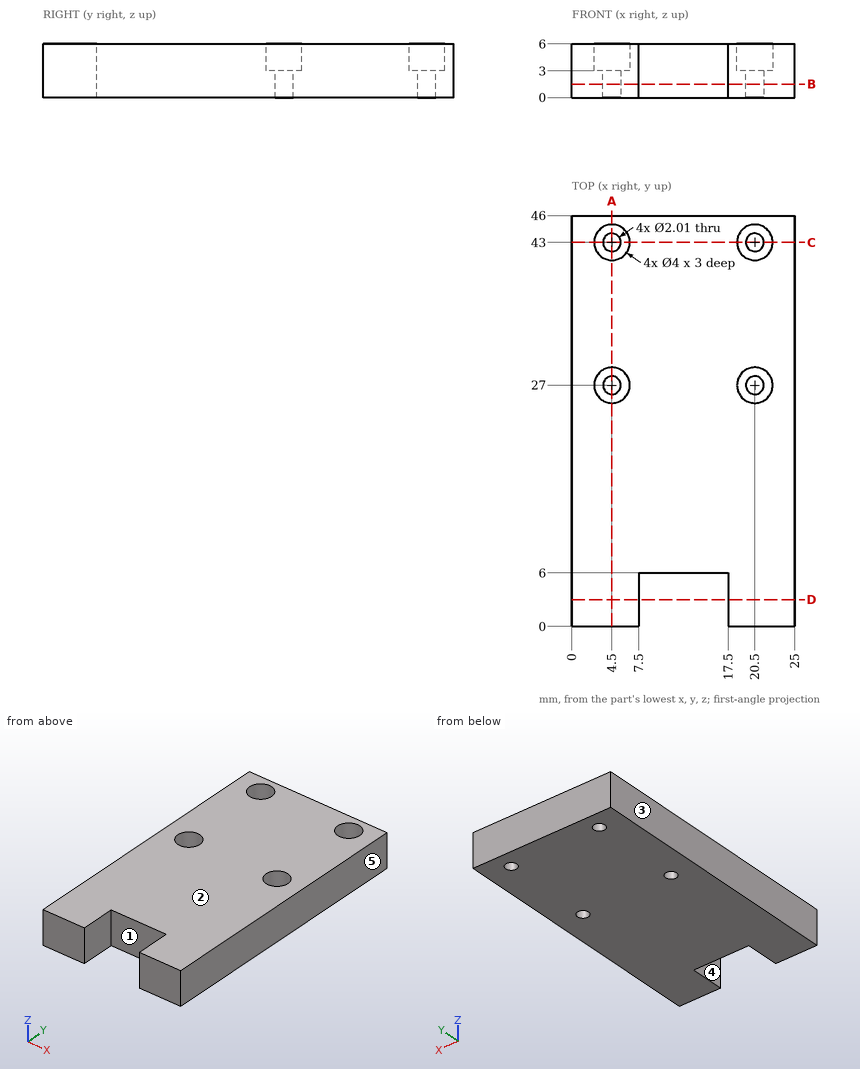
Verification items for this drawing (mm, ordinates from the low corner). A direction names the side the tool comes from. Round coordinates to 2 decimals unless told otherwise and drop trailing zeros. Loops run counter-clockwise (first coordinate to the right, second up) from the corner with the lowest first, then second, coordinate; pieces in that order, holes last. Notation, with made-up numbers: (-26, 19) -> (18, 19) arc R20 cw to (18, 58) -> close; hole circle Ø9 at (81.25, 38.5). An arc over 180 degrees is marked (long way). Write item = value, one per line. Start each with the question number.
1) Gauge pin test, flat ends, axial feed: pin 1 Ø2.5 at (x, y) = (4.5, 43) entering from -Z; pin 2 Ø1.8 at (x, z) = (10.5, 3.5) entering from -Y; pin 3 Ø1.2 at (x, y) = (20.5, 27) entering from +Z; pin 4 Ø2 at (x, y) = (21, 43) entering from +Z. Record the tip position at first contact, or that the pin passes through.
2) Set-up check for the marked faces 4 and 5: record each of +Z, -Z, +X, -X, +Y, -Y from which the full face is reachable in a straight line by a thin tool's end or side.
3) Sectioned sample at D-D, the plane y = 3. Record the cut outline in (x, z), plus the area to 3 significant figures.
4) Sectioned sample at A-A, the plane x = 4.5. Record the cut outline in (y, z) (3 decimals).
5) Sectioned sample at B-B, the plane z = 1.5. Record the cut outline in (x, y) (3 decimals).
6) Sectioned sample at C-C, the plane y = 43. Record the cut outline in (x, z) (3 decimals), plus the area to 3 significant figures.
7) Release check for a two-part mould opening along X. For the marked faces 1, 2 and 3 record: released by +X, released by -X, zero draft, split by the parting line, or undercut.
8) Thickness scan on probe 1 along Y at (x, z) = (20.5, 4.6); probe 2 along X at (y, z) = (43, 1.8) (3 decimals); probe 3 along Y at (x, z) = (16.5, 1.85). Record the ranges inside material, lowest first.
Results are:
q1.pin_1 = 0
q1.pin_2 = 6
q1.pin_3 = through
q1.pin_4 = 3
q2.face_4 = +Z, -Z, -Y
q2.face_5 = +Z, -Z, +X, +Y, -Y
q3.outline = (0, 0) -> (7.5, 0) -> (7.5, 6) -> (0, 6) -> close; (17.5, 0) -> (25, 0) -> (25, 6) -> (17.5, 6) -> close
q3.area = 90.0 mm^2
q4.outline = (0, 0) -> (25.995, 0) -> (25.995, 3) -> (25, 3) -> (25, 6) -> (0, 6) -> close; (28.005, 0) -> (41.995, 0) -> (41.995, 3) -> (41, 3) -> (41, 6) -> (29, 6) -> (29, 3) -> (28.005, 3) -> close; (44.005, 0) -> (46, 0) -> (46, 6) -> (45, 6) -> (45, 3) -> (44.005, 3) -> close
q5.outline = (0, 0) -> (7.5, 0) -> (7.5, 6) -> (17.5, 6) -> (17.5, 0) -> (25, 0) -> (25, 46) -> (0, 46) -> close; hole circle Ø2.01 at (4.5, 27); hole circle Ø2.01 at (4.5, 43); hole circle Ø2.01 at (20.5, 27); hole circle Ø2.01 at (20.5, 43)
q6.outline = (0, 0) -> (3.495, 0) -> (3.495, 3) -> (2.5, 3) -> (2.5, 6) -> (0, 6) -> close; (5.505, 0) -> (19.495, 0) -> (19.495, 3) -> (18.5, 3) -> (18.5, 6) -> (6.5, 6) -> (6.5, 3) -> (5.505, 3) -> close; (21.505, 0) -> (25, 0) -> (25, 6) -> (22.5, 6) -> (22.5, 3) -> (21.505, 3) -> close
q6.area = 114 mm^2
q7.face_1 = undercut
q7.face_2 = zero draft
q7.face_3 = released by -X
q8.probe_1 = 0 to 25, 29 to 41, 45 to 46
q8.probe_2 = 0 to 3.495, 5.505 to 19.495, 21.505 to 25
q8.probe_3 = 6 to 46
